from build123d import *

# Parameters (mm, degrees)
CROQUIS1_W              = 50
CROQUIS1_H              = 10
SALIENTE_EXTRUIR1_DEPTH = 2.5
CORTAR_EXTRUIR1_DEPTH   = 52.23475383
SALIENTE_EXTRUIR2_DEPTH = 5


with BuildPart() as part:
    # Croquis1 → Saliente-Extruir1 (new, symmetric)
    with BuildSketch(Plane(origin=(0, 0, 0), x_dir=(1, 0, 0), z_dir=(0, 1, 0))):
        with Locations((25, 5)):
            Rectangle(CROQUIS1_W, CROQUIS1_H)
    extrude(amount=SALIENTE_EXTRUIR1_DEPTH, both=True)

    # Croquis2 → Cortar-Extruir1 (cut, through all)
    with BuildSketch(Plane(origin=(0, 2.5, 0), x_dir=(1, 0, 0), z_dir=(0, 1, 0))):
        with BuildLine():
            Line((50, 7.5), (37, 7.5))
            ThreePointArc((37, 7.5), (35.585786438, 6.914213562), (35, 5.5))
            Line((35, 5.5), (35, 4.5))
            ThreePointArc((35, 4.5), (35.585786438, 3.085786438), (37, 2.5))
            Line((37, 2.5), (50, 2.5))
            Line((50, 2.5), (50, 7.5))
        make_face()
    extrude(amount=-CORTAR_EXTRUIR1_DEPTH, mode=Mode.SUBTRACT)

    # Croquis3 → Saliente-Extruir2 (add)
    with BuildSketch(Plane(origin=(0, 2.5, 0), x_dir=(1, 0, 0), z_dir=(0, 1, 0))):
        with BuildLine():
            Line((0, 2.5), (-13, 2.5))
            ThreePointArc((-13, 2.5), (-14.414213562, 3.085786438), (-15, 4.5))
            Line((-15, 4.5), (-15, 5.5))
            ThreePointArc((-15, 5.5), (-14.414213562, 6.914213562), (-13, 7.5))
            Line((-13, 7.5), (0, 7.5))
            Line((0, 7.5), (0, 2.5))
        make_face()
    extrude(amount=-SALIENTE_EXTRUIR2_DEPTH)


solid = part.part
Check sheet for the modelled part. Datum: model origin and axes. Units: mm. A direction names the side the tool comes from. Give positions to 0.01 mm unless a question says otherwise; leave off trailing zeros. Write each loop counter-clockwise with the first axis right and the second up, starting at its lowest first coordinate (ties: lowest second). Pieces come first, ordered by that corner, then holes. Notation, with made-up numbers: (-12.5, 53) -> (23.5, 53) arc R31 cw to (23.5, 86) -> close; hole circle Ø6 at (35.5, 42.25). An arc over 180 degrees is marked (long way). One line per item, written item: value. Start each with the question number.
Item 1: Gauge pin test, flat ends, axial feed: pin 1 (1.5 mm diameter, centred on y = -1.5, z = -3.5, fed in from +X); pin 2 (2 mm diameter, centred on y = -1, z = -4.5, fed in from +X); pin 3 (2 mm diameter, centred on y = 0, z = -2, fed in from -X). Record the tip position at first contact, or that the pin passes through.
Item 2: Section check B-B on y = 0.05. Record the cut outline in (x, z), then the cut area to 3 significant figures.
Item 3: Tool access check on faces 5 (the flat face through (17, 2.5, -5)), 6 (the flat face through (44, 0, -7.5)), 7 (the flat face through (25, 0, 0)), 8 (the flat face through (-7, 0, -7.5)), 9 (the flat face through (0, 0, -1)). Record the directions out of +Z, -Z, +X, -X, +Y, -Y that give a thin tool (end or side, any length) a straight path to the whole face; none if there is none.
Item 4: Material ranges on probe 1 along Z at (x, y) = (42.5, 1.7); probe 2 along X at (y, z) = (-1.65, -2); probe 3 along Z at (x, y) = (-4.5, 1.25), recorded low to high. Write a range as from..to.
Item 5: Section check D-D on z = -3.5. Record the cut outline in (x, y).
Item 6: Draft check along Z on faces 1 (the flat face through (50, 0, -1)), 2 (the flat face through (43, 0, -2.5)), 3 (the flat face through (-6, 0, -2.5)), 4 (the cylindrical face through (35.6, 0.04, -6.93)). Enter one of: +Z half, -Z half, draft (parallel to the pull), parting line (faces both ways), or undercut.
Item 7: Section check A-A on x = 41. Record the cut outline in (y, z).
Item 8: Section check C-C on x = -2.5. Record the cut outline in (y, z).
Results list:
1. pin 1: x = 36.03
1. pin 2: x = 35.27
1. pin 3: x = -14.32
2. outline: (-15, -5.5) arc R2 ccw to (-13, -7.5) -> (0, -7.5) -> (0, -10) -> (50, -10) -> (50, -7.5) -> (37, -7.5) arc R2 cw to (35, -5.5) -> (35, -4.5) arc R2 cw to (37, -2.5) -> (50, -2.5) -> (50, 0) -> (0, 0) -> (0, -2.5) -> (-13, -2.5) arc R2 ccw to (-15, -4.5) -> close
2. area: 500 mm²
3. face 5: +Z, -Z, +X, -X, +Y
3. face 6: +X, +Y, -Y
3. face 7: +Z, +X, -X, +Y, -Y
3. face 8: -Z, -X, +Y, -Y
3. face 9: +Z, -X, +Y, -Y
4. probe 1: -10..-7.5, -2.5..0
4. probe 2: 0..50
4. probe 3: -7.5..-2.5
5. outline: (-14.73, -2.5) -> (35.27, -2.5) -> (35.27, 2.5) -> (-14.73, 2.5) -> close
6. face 1: draft
6. face 2: undercut
6. face 3: +Z half
6. face 4: undercut
7. outline: (-2.5, -10) -> (2.5, -10) -> (2.5, -7.5) -> (-2.5, -7.5) -> close; (-2.5, -2.5) -> (2.5, -2.5) -> (2.5, 0) -> (-2.5, 0) -> close
8. outline: (-2.5, -7.5) -> (2.5, -7.5) -> (2.5, -2.5) -> (-2.5, -2.5) -> close
